```python
from build123d import *

# Parameters (mm, degrees)
SKETCH1_W           = 15.6
SKETCH1_H           = 14.6
SKETCH1_R           = 1.7
SKETCH1_W_2         = 3
BOSS_EXTRUDE1_DEPTH = 3.2
SKETCH4_W           = 15.7
SKETCH4_H           = 2.8
SKETCH4_R           = 1.7
BOSS_EXTRUDE3_DEPTH = 4.8


with BuildPart() as part:
    # Sketch1 → Boss-Extrude1 (new body)
    # profile 1 of 4: a face of its own
    with BuildSketch(Plane(origin=(0, 0, 0), x_dir=(1, 0, 0), z_dir=(0, 1, 0))):
        with Locations((-1.5, 0)):
            Rectangle(SKETCH1_W, SKETCH1_H)
        with Locations((-5.8, 0)):
            Circle(SKETCH1_R, mode=Mode.SUBTRACT)
        with Locations((1.6, 0)):
            Circle(SKETCH1_R, mode=Mode.SUBTRACT)
    # profile 2 of 4: a face of its own
    with BuildSketch(Plane(origin=(0, 0, 0), x_dir=(1, 0, 0), z_dir=(0, 1, 0))):
        with Locations((7.8, 0)):
            Rectangle(SKETCH1_W_2, SKETCH1_H)
    # profile 3 of 4: a face of its own
    with BuildSketch(Plane(origin=(0, 0, 0), x_dir=(1, 0, 0), z_dir=(0, 1, 0))):
        with Locations((1.6, 0)):
            Circle(SKETCH1_R)
    # profile 4 of 4: a face of its own
    with BuildSketch(Plane(origin=(0, 0, 0), x_dir=(1, 0, 0), z_dir=(0, 1, 0))):
        with Locations((-5.8, 0)):
            Circle(SKETCH1_R)
    extrude(amount=BOSS_EXTRUDE1_DEPTH)

    # Sketch4 → Boss-Extrude3 (add)
    with BuildSketch(Plane(origin=(0, 3.2, 0), x_dir=(1, 0, 0), z_dir=(0, 1, 0))):
        with Locations((-1.45, 5.9)):
            Rectangle(SKETCH4_W, SKETCH4_H)
        Polygon((6.4, -4.5), (6.4, -7.3), (9.3, -7.3), (9.3, 7.3), (6.4, 7.3), (6.4, 4.5), align=None)
        with Locations(Location((-5.7, 0, 0), (0, 0, 270))):
            Circle(SKETCH4_R)
        with Locations(Location((1.7, 0, 0), (0, 0, 270))):
            Circle(SKETCH4_R)
        with Locations((-1.45, -5.9)):
            Rectangle(SKETCH4_W, SKETCH4_H)
    extrude(amount=BOSS_EXTRUDE3_DEPTH)


solid = part.part
```
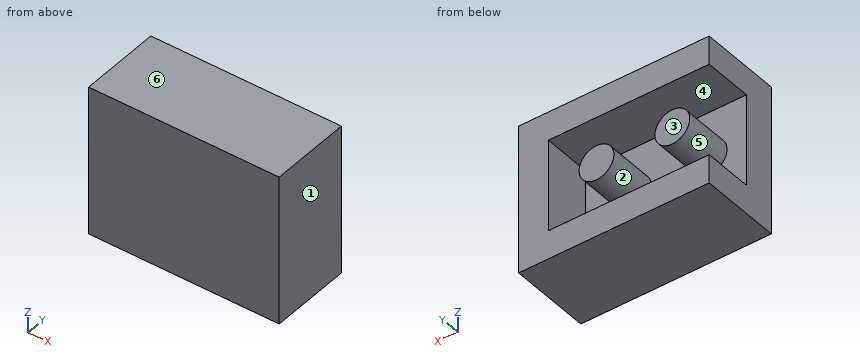
Source: CAD feature listing. Evaluate the final solid. Frame: model axes, mm. Face numbers are marked on the shaded views. A direction names the side the tool comes from. Coordinates: 2 decimals unless noted, no trailing zeros. Order: outer loops, then holes, each group sorted by start corner. A loop starts at its lowest first (then second) coordinate and runs counter-clockwise, first axis right, second up. Notation, with made-up numbers: (87, 22) - (106, 22) arc R15 cw to (106, 38) - close; hole circle Ø2 at (18.5, 2.5). An arc over 180 degrees is marked (long way). One line per item, written item: value.
1) Mould query, pull axis X, two halves, no side actions, for the marked faces 1, 2 and 3. Classes: released by +X, released by -X, zero draft, split by the parting line, or undercut.
Computed values:
face 1: released by +X
face 2: undercut
face 3: zero draft
2) Cut plane D-D on z = -2. Output: boundary loops of the cut face in (x, y), plus the area to 3 significant figures.
Computed values:
outline: (-9.3, 0) - (9.3, 0) - (9.3, 8) - (6.4, 8) - (6.4, 3.2) - (-9.3, 3.2) - close
area: 73.4 mm^2
3) Cut plane A-A on x = -2.25. Output: boundary loops of the cut face in (y, z).
Computed values:
outline: (0, -7.3) - (8, -7.3) - (8, -4.5) - (3.2, -4.5) - (3.2, 4.5) - (8, 4.5) - (8, 7.3) - (0, 7.3) - close
4) Contact query for flat-ended pins moving along their axis: pin 1 (1.4 mm diameter, centred on y = 4.5, z = 1, fed in from -X); pin 2 (2 mm diameter, centred on x = -3, z = 3, fed in from -Y). Output: stop coordinate, or through.
Computed values:
pin 1: stops at x = -7.37
pin 2: stops at y = 0
5) Cut plane C-C on x = -5.7. Output: boundary loops of the cut face in (y, z), plus the area to 3 significant figures.
Computed values:
outline: (0, -7.3) - (8, -7.3) - (8, -4.5) - (3.2, -4.5) - (3.2, -1.7) - (8, -1.7) - (8, 1.7) - (3.2, 1.7) - (3.2, 4.5) - (8, 4.5) - (8, 7.3) - (0, 7.3) - close
area: 89.9 mm^2
6) Cut plane B-B on z = 0. Output: boundary loops of the cut face in (x, y), plus the area to 3 significant figures.
Computed values:
outline: (-9.3, 0) - (9.3, 0) - (9.3, 8) - (6.4, 8) - (6.4, 3.2) - (3.4, 3.2) - (3.4, 8) - (0, 8) - (0, 3.2) - (-4, 3.2) - (-4, 8) - (-7.4, 8) - (-7.4, 3.2) - (-9.3, 3.2) - close
area: 106 mm^2
7) Ray query, line 1 (Z direction, x = -4.25, y = 6); line 2 (Z direction, x = -6.75, y = 3.5); line 3 (Y direction, x = 2.5, z = 2.5). Return the intervals inside material, ascending. Write a range as [from, to].
Computed values:
line 1: z = [-7.3, -4.5], [-0.89, 0.89], [4.5, 7.3]
line 2: z = [-7.3, -4.5], [-1.34, 1.34], [4.5, 7.3]
line 3: y = [0, 3.2]
8) Reachability of the marked faces 4, 5 and 6 from +Z, -Z, +X, -X, +Y, -Y: full face, straight path, thin tool, end or side. Return the list, or none.
Computed values:
face 4: -X, +Y
face 5: +Y
face 6: +Z, +X, -X, +Y, -Y
